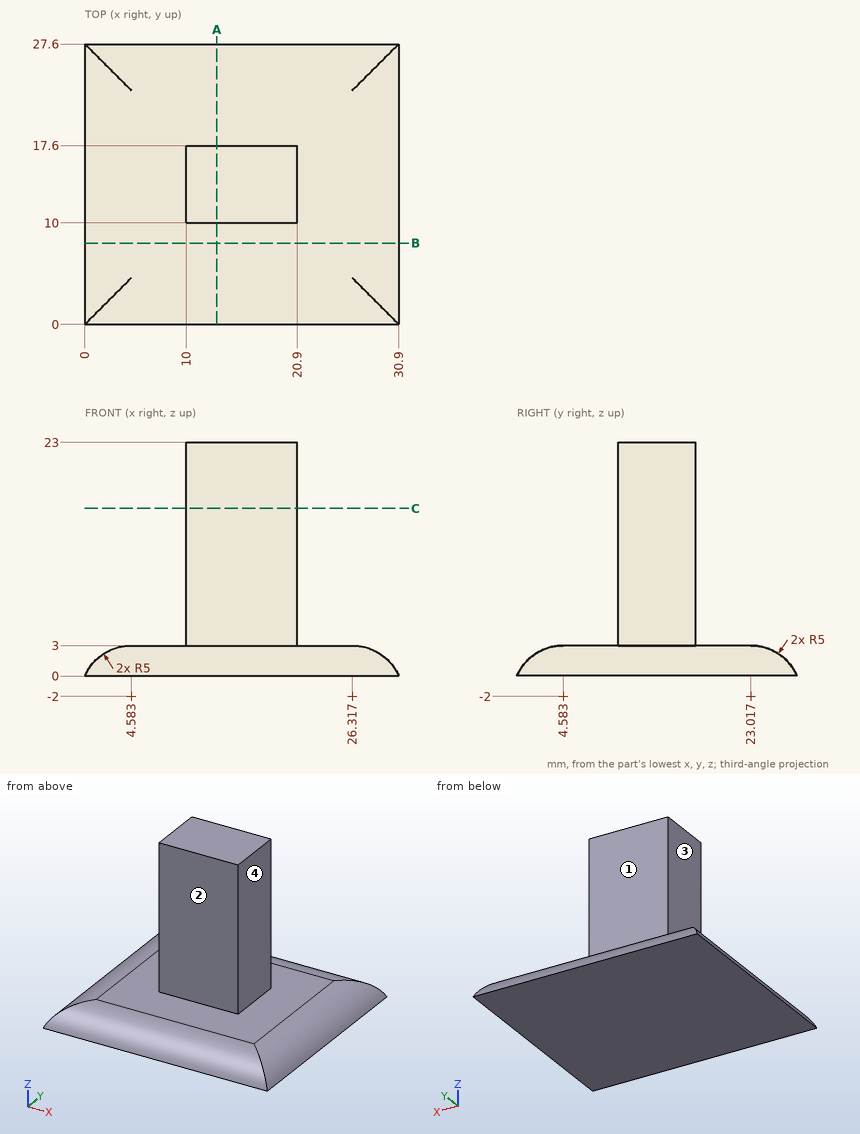
Source: three-view drawing plus pictorial views. Frame: mm from the lowest corner of the part. A direction names the side the tool comes from. Round coordinates to 2 decimals unless told otherwise and drop trailing zeros. Order: outer loops, then holes, each group sorted by start corner. A loop starts at its lowest first (then second) coordinate and runs counter-clockwise, first axis right, second up. Notation, with made-up numbers: (36.25, 29.25) - (83.25, 29.25) arc R19 cw to (83.25, 50.25) - close; hole circle Ø5 at (-14.5, 78.5). An arc over 180 degrees is marked (long way). Answer in a Markdown table with one row per item.
Item 1: Section query B-B (y = 8). Return the cut outline in (x, z).
Model answer:
| item | result |
|---|---|
| outline | (0, 0) - (30.9, 0) arc R5 ccw to (26.32, 3) - (4.58, 3) arc R5 ccw to start |
Item 2: Section query C-C (z = 16.5). Return the cut outline in (x, y).
Model answer:
| item | result |
|---|---|
| outline | (10, 10) - (20.9, 10) - (20.9, 17.6) - (10, 17.6) - close |
Item 3: Line query: line 1 (X direction, y = 12, z = 8); line 2 (Y direction, x = 18, z = 18); line 3 (Z direction, x = 7.5, y = 8.25). Output: solid intervals per line, ascending.
Model answer:
| item | result |
|---|---|
| line 1 | x = 10 to 20.9 |
| line 2 | y = 10 to 17.6 |
| line 3 | z = 0 to 3 |
Item 4: Reachability of the marked faces 1, 2, 3 and 4 from +Z, -Z, +X, -X, +Y, -Y: full face, straight path, thin tool, end or side. Return the list, or none.
Model answer:
| item | result |
|---|---|
| face 1 | +Z, +X, -X, +Y |
| face 2 | +Z, +X, -X, -Y |
| face 3 | +Z, -X, +Y, -Y |
| face 4 | +Z, +X, +Y, -Y |
Item 5: Section query A-A (x = 13). Return the cut outline in (y, z).
Model answer:
| item | result |
|---|---|
| outline | (0, 0) - (27.6, 0) arc R5 ccw to (23.02, 3) - (17.6, 3) - (17.6, 23) - (10, 23) - (10, 3) - (4.58, 3) arc R5 ccw to start |
Item 6: Pin query (flat end, axial travel): pin 1 (8.5 mm diameter, centred on x = 18, z = 16, fed in from -Y); pin 2 (8 mm diameter, centred on y = 19.5, z = 3, fed in from -X); pin 3 (2.5 mm diameter, centred on y = 13, z = 11.5, fed in from -X); pin 4 (8.5 mm diameter, centred on y = 12.5, z = 14, fed in from +X). Return the tip coordinate at first contact, or that it passes through.
Model answer:
| item | result |
|---|---|
| pin 1 | stops at y = 10 |
| pin 2 | stops at x = 0 |
| pin 3 | stops at x = 10 |
| pin 4 | stops at x = 20.9 |
